Geometry check sheet. Reference: the model listing, model coordinates, mm. Face numbers are marked on the shaded views. A direction names the side the tool comes from. Coordinates: 2 decimals unless noted, no trailing zeros. Loops run counter-clockwise (first coordinate to the right, second up) from the corner with the lowest first, then second, coordinate; pieces in that order, holes last.
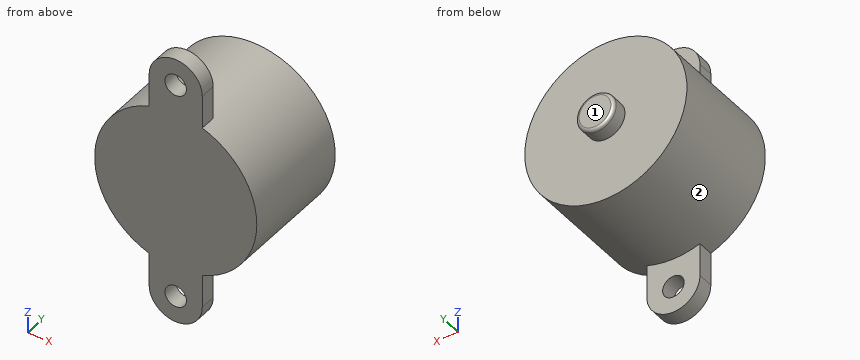
from build123d import *

# Parameters (mm, degrees)
SKETCH1_R           = 12.75
BOSS_EXTRUDE1_DEPTH = 18
SKETCH2_R           = 3
BOSS_EXTRUDE2_DEPTH = 2.5
FILLET1_R           = 0.5
SKETCH3_R           = 1.69339008
BOSS_EXTRUDE3_DEPTH = 2.5


with BuildPart() as part:
    # Sketch1 → Boss-Extrude1 (new body)
    with BuildSketch(Plane(origin=(0, 0, 0), x_dir=(1, 0, 0), z_dir=(0, 1, 0))):
        Circle(SKETCH1_R)
    extrude(amount=BOSS_EXTRUDE1_DEPTH)

    # Sketch2 → Boss-Extrude2 (add)
    with BuildSketch(Plane(origin=(0, 18, 0), x_dir=(1, 0, 0), z_dir=(0, 1, 0))):
        Circle(SKETCH2_R)
    extrude(amount=BOSS_EXTRUDE2_DEPTH)

    # Fillet1
    fillet1_edges = [part.edges().sort_by_distance(p)[0] for p in [
        (-3, 20.5, 0),
    ]]
    fillet(fillet1_edges, radius=FILLET1_R)

    # Sketch3 → Boss-Extrude3 (add)
    with BuildSketch(Plane(origin=(0, 0, 0), x_dir=(1, 0, 0), z_dir=(0, 1, 0))):
        with BuildLine():
            Line((4.175, 12.047069146), (4.175, 17.252375634))
            ThreePointArc((4.175, 17.252375634), (0, 21.427375634), (-4.175, 17.252375634))
            Line((-4.175, 17.252375634), (-4.175, 12.047069146))
            Line((-4.175, 12.047069146), (4.175, 12.047069146))
        make_face()
        with Locations((0, 17.252375634)):
            Circle(SKETCH3_R, mode=Mode.SUBTRACT)
    boss_extrude3 = extrude(amount=BOSS_EXTRUDE3_DEPTH)

    # Mirror1: Boss-Extrude3 across plane
    add(boss_extrude3.mirror(Plane.XY))


solid = part.part
1) Depth check by flat-ended pin: pin 1 (6 mm diameter, centred on x = -2, y = 13.5, fed in from -Z); pin 2 (2 mm diameter, centred on x = -5, y = 16, fed in from -Z); pin 3 (3 mm diameter, centred on x = 6.5, y = 3, fed in from -Z); pin 4 (2.5 mm diameter, centred on x = 0, z = -17.25, fed in from +Y) (1 decimal). Enter the tip coordinate at first touch or a pass-through.
Data:
pin 1: stops at z = -12.75
pin 2: stops at z = -12.11
pin 3: stops at z = -11.73
pin 4: passes through
2) Section check D-D on x = 7. Record the cut outline in (y, z), and give its area (3 significant figures).
Data:
outline: (0, -10.66) - (18, -10.66) - (18, 10.66) - (0, 10.66) - close
area: 384 mm2
3) Section check A-A on x = 0. Record the cut outline in (y, z), and give its area (3 significant figures).
Data:
outline: (0, -21.43) - (2.5, -21.43) - (2.5, -18.95) - (0, -18.95) - close; (0, -15.56) - (2.5, -15.56) - (2.5, -12.75) - (18, -12.75) - (18, -3) - (20, -3) arc R0.5 ccw to (20.5, -2.5) - (20.5, 2.5) arc R0.5 ccw to (20, 3) - (18, 3) - (18, 12.75) - (2.5, 12.75) - (2.5, 15.56) - (0, 15.56) - close; (0, 18.95) - (2.5, 18.95) - (2.5, 21.43) - (0, 21.43) - close
area: 500 mm2
4) Access from +Z, -Z, +X, -X, +Y, -Y to the whole of each face (thin tool, end or side, straight path). Record for the marked faces 1 and 2.
Data:
face 1: +Z, -Z, +X, -X, +Y
face 2: +Y
5) Material ranges on probe 1 along Z at (x, y) = (0, 1.85); probe 2 along X at (y, z) = (2, -15) (3 decimals); probe 3 along Y at (x, z) = (-6.25, 2), recorded low to high.
Data:
probe 1: z = -21.43 to -18.95, -15.56 to 15.56, 18.95 to 21.43
probe 2: x = -4.175 to 4.175
probe 3: y = 0 to 18
6) Section check C-C on y = 13. Record the cut outline in (x, z).
Data:
outline: circle Ø25.5 at (0, 0)
7) Section check B-B on z = 0. Record the cut outline in (x, y).
Data:
outline: (-12.75, 0) - (12.75, 0) - (12.75, 18) - (3, 18) - (3, 20) arc R0.5 ccw to (2.5, 20.5) - (-2.5, 20.5) arc R0.5 ccw to (-3, 20) - (-3, 18) - (-12.75, 18) - close
